Here's how the part is built. I have some questions about the finished solid (model axes, mm). Face numbers are marked on the shaded views. Give positions to 0.01 mm unless a question says otherwise; leave off trailing zeros. Loops run counter-clockwise (first coordinate to the right, second up) from the corner with the lowest first, then second, coordinate; pieces in that order, holes last.
Q1. Suppose I cut it at C-C (x = 167). List the corners of the cut face in (y, z) for me.
Q2. I'm going to push flat-ended pins straight in: P1, Ø1, axis at x = 269, y = 56.5, coming from the -Z side; P2, Ø1, axis at x = 267.5, y = -110.5, coming from the +Z side; P3, Ø15, axis at x = -334.5, z = -818, coming from the +Y side. Where does each tip first touch, or does it pass through?
Q3. Thinking about a two-plate mould opening in X: for the marked faces 1 and 2, which applies, pulls with the +X half, pulls with the -X half, needs draft (parallel to the pull), parting line crosses it, or undercut?
Q4. Suppose I cut it at D-D (y = 126.5). List the corners of the cut face in (x, z) for me, and give its area (3 significant figures).
Q5. Suppose I cut it at B-B (y = -117). List the corners of the cut face in (x, z) for me.
Q6. Suppose I cut it at A-A (z = -307.5). List the corners of the cut face in (x, y) for me, and give its area (3 significant figures).
Q7. I need wall thicknesses on probe 1 along Y at (x, z) = (322, -163); probe 2 along Z at (x, y) = (-311, -31); probe 3 along Z at (x, y) = (-128, 173). Which ranges of each line are inside material? Lowest first, please.
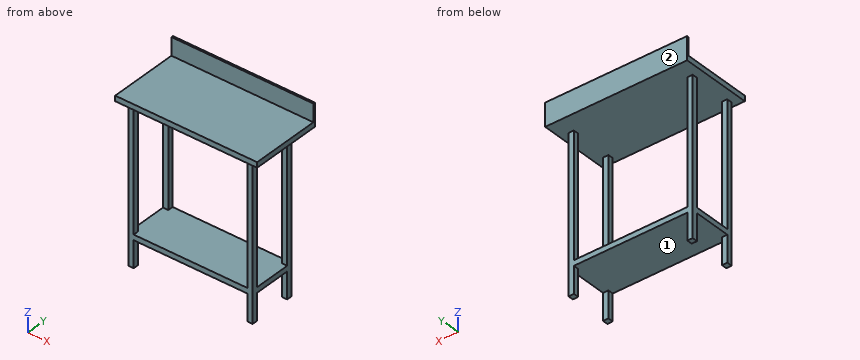
```python
from build123d import *

# Parameters (mm, degrees)
F0_W          = 800
F0_H          = 400
F1_DEPTH      = 30
F2_W          = 800
F2_H          = 10
F3_DEPTH      = 100
F4_W          = 30
F4_H          = 30
F5_DEPTH      = 875
F6_W          = 700
F6_H          = 30
F7_DEPTH      = 170
F7_DEPTH_BACK = 100


with BuildPart() as f1:
    # F0 (on Top) → F1 (new body)
    with BuildSketch(Plane.XY):
        Rectangle(F0_W, F0_H)
    extrude(amount=F1_DEPTH)

    # F2 (on face) → F3 (join)
    with BuildSketch(Plane.XY.offset(30)):
        with Locations((0, 195)):
            Rectangle(F2_W, F2_H)
    extrude(amount=F3_DEPTH)

    # F4 (on face) → F5 (join)
    with BuildSketch(Plane(origin=(0, 0, 0), x_dir=(1, 0, 0), z_dir=(0, 0, -1))):
        with Locations((335, 155)):
            Rectangle(F4_W, F4_H)
        with Locations((335, -85)):
            Rectangle(F4_W, F4_H)
        with Locations((-335, 155)):
            Rectangle(F4_W, F4_H)
        with Locations((-335, -85)):
            Rectangle(F4_W, F4_H)
    extrude(amount=F5_DEPTH)

    # F6 (on Front) → F7 (join, two sides)
    with BuildSketch(Plane.XZ) as f7_sk:
        with Locations((0, -710)):
            Rectangle(F6_W, F6_H)
    extrude(amount=F7_DEPTH)
    extrude(f7_sk.sketch, amount=-F7_DEPTH_BACK)


solid = f1.part
```
Solutions:
1. outline: (-200, 0) - (200, 0) - (200, 130) - (190, 130) - (190, 30) - (-200, 30) - close; (-170, -725) - (100, -725) - (100, -695) - (-170, -695) - close
2. P1: stops at z = -725
2. P2: stops at z = 30
2. P3: stops at y = 100
3. face 1: undercut
3. face 2: needs draft
4. outline: (-400, 0) - (400, 0) - (400, 30) - (-400, 30) - close
4. area: 24,000 mm2
5. outline: (-400, 0) - (400, 0) - (400, 30) - (-400, 30) - close; (-350, -725) - (350, -725) - (350, -695) - (-350, -695) - close
6. outline: (-350, -170) - (-320, -170) - (-320, -140) - (-350, -140) - close; (-350, 70) - (-320, 70) - (-320, 100) - (-350, 100) - close; (320, -170) - (350, -170) - (350, -140) - (320, -140) - close; (320, 70) - (350, 70) - (350, 100) - (320, 100) - close
6. area: 3,600 mm2
7. probe 1: y = -170 to -140, 70 to 100
7. probe 2: z = -725 to -695, 0 to 30
7. probe 3: z = 0 to 30
